from build123d import *

# Parameters (mm, degrees)
SKETCH1_R           = 30.5
BOSS_EXTRUDE1_DEPTH = 5
SKETCH2_R           = 15.75
CUT_EXTRUDE1_DEPTH  = 2.5
SKETCH3_R           = 15.75
BOSS_EXTRUDE2_DEPTH = 2.5
SKETCH4_R           = 3.25
CUT_EXTRUDE2_DEPTH  = 5.08
SKETCH5_R           = 3.25
CUT_EXTRUDE3_DEPTH  = 5.08
SKETCH6_R           = 3.25
CUT_EXTRUDE4_DEPTH  = 5.08
BOSS_EXTRUDE3_DEPTH = 5.08
SKETCH8_W           = 25.4
SKETCH8_H           = 6.35
BOSS_EXTRUDE4_DEPTH = 25.4
SKETCH9_W           = 25.4
SKETCH9_H           = 3.81
BOSS_EXTRUDE5_DEPTH = 25.4
SKETCH10_R          = 3.302
CUT_EXTRUDE5_DEPTH  = 7.62
SKETCH12_R          = 4.826
CUT_EXTRUDE6_DEPTH  = 2.54


with BuildPart() as part:
    # Sketch1 → Boss-Extrude1 (new body)
    with BuildSketch(Plane(origin=(0, 0, 0), x_dir=(1, 0, 0), z_dir=(0, 1, 0))):
        with Locations(Location((0, 0, 0), (0, 0, 270))):
            Circle(SKETCH1_R)
    extrude(amount=BOSS_EXTRUDE1_DEPTH)

    # Sketch2 → Cut-Extrude1 (cut)
    with BuildSketch(Plane(origin=(0, 5, 0), x_dir=(1, 0, 0), z_dir=(0, 1, 0))):
        with Locations(Location((0, 0, 0), (0, 0, 270))):
            Circle(SKETCH2_R)
    extrude(amount=-CUT_EXTRUDE1_DEPTH, mode=Mode.SUBTRACT)

    # Sketch3 → Boss-Extrude2 (add)
    with BuildSketch(Plane.XZ):
        with Locations(Location((0, 0, 0), (0, 0, 90))):
            Circle(SKETCH3_R)
    extrude(amount=BOSS_EXTRUDE2_DEPTH)

    # Sketch4 → Cut-Extrude2 (cut)
    with BuildSketch(Plane(origin=(0, 0, 0), x_dir=(-1, 0, 0), z_dir=(0, -1, 0))):
        with Locations(Location((0, 25, 0), (0, 0, 90))):
            Circle(SKETCH4_R)
    extrude(amount=-CUT_EXTRUDE2_DEPTH, mode=Mode.SUBTRACT)

    # Sketch5 → Cut-Extrude3 (cut)
    with BuildSketch(Plane.XZ):
        with Locations(Location((0, 25, 0), (0, 0, 270))):
            Circle(SKETCH5_R)
    extrude(amount=-CUT_EXTRUDE3_DEPTH, mode=Mode.SUBTRACT)

    # Sketch6 → Cut-Extrude4 (cut)
    with BuildSketch(Plane.XZ):
        with Locations(Location((17.674476483, 17.680862, 0), (0, 0, 270))):
            Circle(SKETCH6_R)
    extrude(amount=-CUT_EXTRUDE4_DEPTH, mode=Mode.SUBTRACT)

    # Sketch7 → Boss-Extrude3 (add)
    with BuildSketch(Plane.XZ):
        with BuildLine():
            ThreePointArc((12.7, -27.73012802), (6.499272859, -29.79948745), (0, -30.5))
            ThreePointArc((0, -30.5), (-6.499272859, -29.79948745), (-12.7, -27.73012802))
            Line((-12.7, -27.73012802), (-12.7, -40.43012802))
            Line((-12.7, -40.43012802), (12.7, -40.43012802))
            Line((12.7, -40.43012802), (12.7, -27.73012802))
        make_face()
    extrude(amount=-BOSS_EXTRUDE3_DEPTH)

    # Sketch8 → Boss-Extrude4 (add)
    with BuildSketch(Plane(origin=(0, 5.08, 0), x_dir=(1, 0, 0), z_dir=(0, 1, 0))):
        with Locations((0, 37.25512802)):
            Rectangle(SKETCH8_W, SKETCH8_H)
    extrude(amount=BOSS_EXTRUDE4_DEPTH)

    # Sketch9 → Boss-Extrude5 (add)
    with BuildSketch(Plane(origin=(0, 0, -40.43012802), x_dir=(-1, 0, 0), z_dir=(0, 0, -1))):
        with Locations((0, 8.255)):
            Rectangle(SKETCH9_W, SKETCH9_H)
    extrude(amount=BOSS_EXTRUDE5_DEPTH)

    # Sketch10 → Cut-Extrude5 (cut)
    with BuildSketch(Plane(origin=(0, 0, -40.43012802), x_dir=(-1, 0, 0), z_dir=(0, 0, -1))):
        with Locations((0, 20.32)):
            Circle(SKETCH10_R)
    extrude(amount=-CUT_EXTRUDE5_DEPTH, mode=Mode.SUBTRACT)

    # Sketch12 → Cut-Extrude6 (cut)
    with BuildSketch(Plane.XY.offset(-34.08012802)):
        with Locations((0, 20.32)):
            Circle(SKETCH12_R)
    extrude(amount=-CUT_EXTRUDE6_DEPTH, mode=Mode.SUBTRACT)


solid = part.part
The model under review builds one solid part; all positions refer to its coordinate system, in mm. A direction names the side the tool comes from. Round coordinates to 2 decimals unless told otherwise and drop trailing zeros. Write each loop counter-clockwise with the first axis right and the second up, starting at its lowest first coordinate (ties: lowest second). Pieces come first, ordered by that corner, then holes. Notation, with made-up numbers: M -8,-33.75 L 8,-33.75 A20 cw 8,-4.75 Z; hole C 86.5,46.5 d10. An arc over 180 degrees is marked long. Use a Markdown table: item, result. Add a question column.
Q1. We need section A-A, the plane y = 20.32. State the section outline as (x, z) points.
Q2. Machinability: for faces 1 (the face through (15.616, 3.768, -2.05)), 2 (the face through (0, 5.08, -32)), 3 (the face through (3, 18, -40.43)), 4 (the face through (0, 3, -40.43)), which of the approach directions +Z, -Z, +X, -X, +Y, -Y give a long, thin tool a straight path to every point of the face, cutting with its end or side? Answer none if there is none.
Q3. We need section D-D, the plane z = -58.5. State the section outline as (x, y) points, plus the area to 3 significant figures.
Q4. We need section B-B, the plane z = 0. State the section outline as (x, y) points, plus the area to 3 significant figures.
Q5. The part is to be moulded in two halves that separate along Z. For faces 5 (the face through (0, 15, -34.08)), 6 (the face through (-0.628, 25.105, -35.332)), 7 (the face through (20.897, 2.465, 18.104)), say which applies: pulls with the +Z half, pulls with the -Z half, needs draft (parallel to the pull), parting line crosses it, or undercut.
Q6. Insertion check: pin 1 (20.5 mm diameter, centred on x = -5.5, z = -59, fed in from +Y); pin 2 (9 mm diameter, centred on y = 9, z = -56, fed in from +X); pin 3 (2 mm diameter, centred on x = 9.5, y = 19.5, fed in from +Z); pin 4 (8 mm diameter, centred on x = 18.5, z = -42, fed in from +Y). Each pin has a flat end and moves straight along its axis. Give the tip position at first contact, or say it passes through.
Q7. We need section C-C, the plane z = -25. State the section outline as (x, y) points, plus the area to 3 significant figures.
Q8. To check wall thickness, follow line 1 (X direction, y = 3.9, z = 0); line 2 (Y direction, x = -7.5, z = -56.5); line 3 (Z direction, x = 8.5, y = 7). State the ranges of each line that lie inside material, in increasing order.
Findings below:
| question | item | result |
|---|---|---|
| 1 | outline | M -12.7,-40.43 L -3.3,-40.43 L -3.3,-36.62 L -4.83,-36.62 L -4.83,-34.08 L -12.7,-34.08 Z; M 3.3,-40.43 L 12.7,-40.43 L 12.7,-34.08 L 4.83,-34.08 L 4.83,-36.62 L 3.3,-36.62 Z |
| 2 | face 1 | +Y |
| 2 | face 2 | +Z, +X, -X, +Y |
| 2 | face 3 | -Z, +X, -X, +Y |
| 2 | face 4 | -Z, +X, -X, -Y |
| 3 | outline | M -12.7,6.35 L 12.7,6.35 L 12.7,10.16 L -12.7,10.16 Z |
| 3 | area | 96.8 mm² |
| 4 | outline | M -30.5,0 L -15.75,0 L -15.75,-2.5 L 15.75,-2.5 L 15.75,0 L 30.5,0 L 30.5,5 L 15.75,5 L 15.75,2.5 L -15.75,2.5 L -15.75,5 L -30.5,5 Z |
| 4 | area | 305 mm² |
| 5 | face 5 | pulls with the +Z half |
| 5 | face 6 | needs draft |
| 5 | face 7 | undercut |
| 6 | pin 1 | stops at y = 10.16 |
| 6 | pin 2 | stops at x = 12.7 |
| 6 | pin 3 | stops at z = -34.08 |
| 6 | pin 4 | passes through |
| 7 | outline | M -17.47,0 L -3.25,0 L -3.25,5 L -17.47,5 Z; M 3.25,0 L 17.47,0 L 17.47,5 L 3.25,5 Z |
| 7 | area | 142 mm² |
| 8 | line 1 | x = -30.5 to -15.75, 15.75 to 30.5 |
| 8 | line 2 | y = 6.35 to 10.16 |
| 8 | line 3 | z = -65.83 to -34.08 |
